```python
from build123d import *

# Parameters (mm, degrees)
SKETCH2_R           = 22.225
BOSS_EXTRUDE1_DEPTH = 7
SKETCH3_R           = 12.7
CUT_EXTRUDE1_DEPTH  = 33.200951073


with BuildPart() as part:
    # Sketch2 → Boss-Extrude1 (new body)
    with BuildSketch(Plane.XY):
        Circle(SKETCH2_R)
    extrude(amount=BOSS_EXTRUDE1_DEPTH)

    # Sketch3 → Cut-Extrude1 (cut, through all)
    with BuildSketch(Plane.XY.offset(7)):
        Circle(SKETCH3_R)
    extrude(amount=-CUT_EXTRUDE1_DEPTH, mode=Mode.SUBTRACT)

    # Sketch4 → Cut-Revolve1 (revolve, cut)
    with BuildSketch(Plane(origin=(0, 0, 0), x_dir=(1, 0, 0), z_dir=(0, 1, 0)), mode=Mode.PRIVATE) as cut_revolve1_sk:
        with BuildLine():
            Line((-18.706967285, -7), (0, -7))
            Line((0, -7), (0, -0.761013597))
            Line((0, -0.761013597), (-12.7, -0.761013597))
            ThreePointArc((-12.7, -0.761013597), (-16.010329052, -3.585072538), (-18.706967285, -7))
        make_face()
    revolve(cut_revolve1_sk.sketch.rotate(Axis((0, 0, -16.764248705), (0, 0, 1)), 180), axis=Axis((0, 0, -16.764248705), (0, 0, 1)), mode=Mode.SUBTRACT)


solid = part.part
```
Can you work these out from the model? Positions are in its coordinate system, mm. Coordinates: 2 decimals unless noted, no trailing zeros. Write each loop counter-clockwise with the first axis right and the second up, starting at its lowest first coordinate (ties: lowest second). Pieces come first, ordered by that corner, then holes. Notation, with made-up numbers: (47.25, 48) - (74.25, 48) arc R9 cw to (74.25, 57) - close; hole circle Ø7 at (57, 47). An arc over 180 degrees is marked (long way). Return JSON: item names as keys, results as strings.
Q1. If we section it at C-C (z = 3): Please give me the cut outline in (x, y) (3 decimals), then the cut area to 3 significant figures.
Computed values:
{"outline": "circle Ø44.45 at (0, 0); hole circle Ø30.851 at (0, 0)", "area": "804 mm2"}
Q2. If we section it at A-A (x = 0): Please give me the cut outline in (y, z) (3 decimals).
Computed values:
{"outline": "(-22.225, 0) - (-12.7, 0) - (-12.7, 0.761) arc R22.225 cw to (-18.707, 7) - (-22.225, 7) - close; (12.7, 0) - (22.225, 0) - (22.225, 7) - (18.707, 7) arc R22.225 cw to (12.7, 0.761) - close"}
Q3. I'm going to push flat-ended pins straight in: pin 1 Ø8 at (x, y) = (-3.5, -3.5) entering from -Z; pin 2 Ø2 at (x, z) = (15.5, 5.5) entering from +Y; pin 3 Ø1.5 at (x, z) = (-7.5, 2.5) entering from -Y; pin 4 Ø10 at (x, y) = (14.5, -10) entering from +Z. Where does each tip first touch, or does it pass through?
Computed values:
{"pin 1": "passes through", "pin 2": "stops at y = 16.84", "pin 3": "stops at y = -21.18", "pin 4": "stops at z = 7"}
Q4. Thinking about a two-plate mould opening in Y: for faces 1 (the cylindrical face through (21.199, 6.676, 3.451)), 2 (the flat face through (-12, -15, 7)), 3 (the cylindrical face through (-2.75, -12.4, 0.39)), which applies, +Y half, -Y half, draft (parallel to the pull), parting line (faces both ways), or undercut?
Computed values:
{"face 1": "parting line", "face 2": "draft", "face 3": "undercut"}
Q5. Please list where these lines run through material, in increasing order: L1, parallel to Y at x = 0, z = 0.5 (3 decimals); L2, parallel to X at y = 12.5, z = 6.75; L3, parallel to X at y = -3, z = 1. Write a range as from..to.
Computed values:
{"L1": "y = -22.225..-12.7, 12.7..22.225", "L2": "x = -18.38..-13.7, 13.7..18.38", "L3": "x = -22.02..-12.69, 12.69..22.02"}
Q6. If we section it at D-D (x = -16): Please give me the cut outline in (y, z).
Computed values:
{"outline": "(-15.43, 0) - (15.43, 0) - (15.43, 7) - (9.69, 7) arc R15.43 cw to (-9.69, 7) - (-15.43, 7) - close"}
